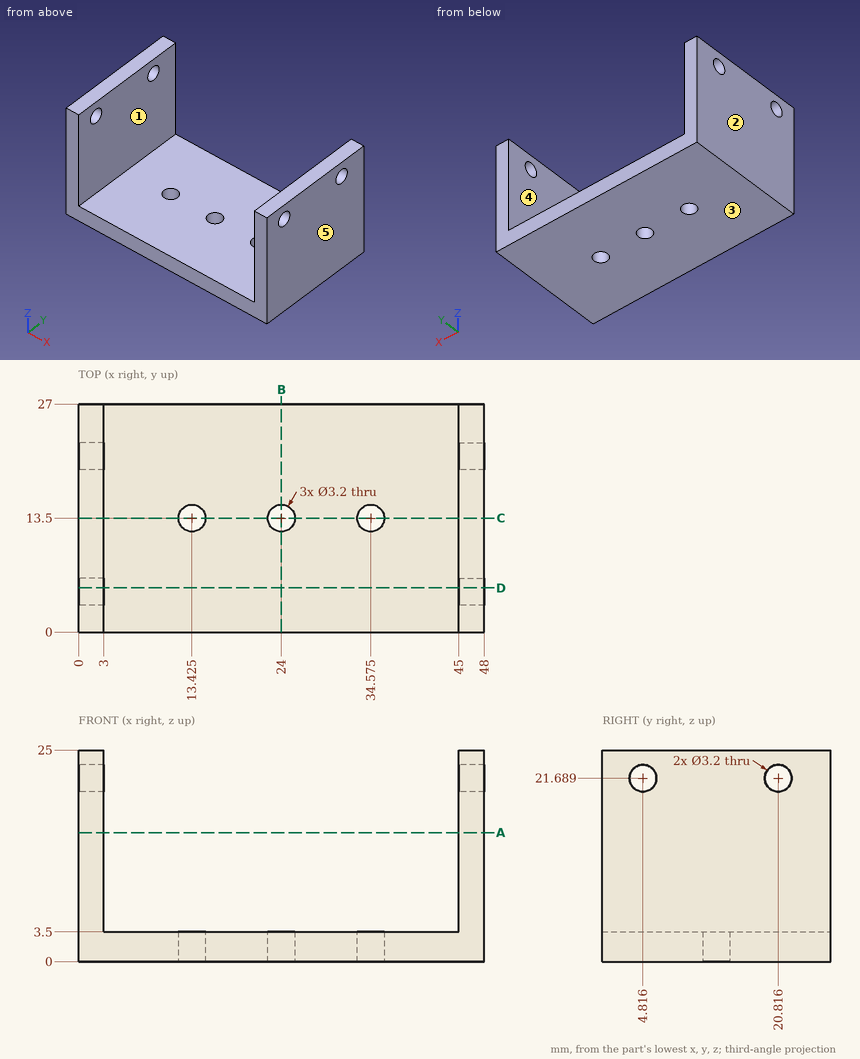
The drawing under review shows one solid part. Ordinate dimensions are in mm from its lowest x, y, z. A direction names the side the tool comes from. Give positions to 0.01 mm unless a question says otherwise; leave off trailing zeros. Loops run counter-clockwise (first coordinate to the right, second up) from the corner with the lowest first, then second, coordinate; pieces in that order, holes last. Notation, with made-up numbers: M 26.5,-9 L 41.5,-9 A9 ccw 41.5,-5 Z; hole C -4,79 d6. An arc over 180 degrees is marked long. Return JSON: item names as keys, results as strings. Group by question number.
Item 1: We need section D-D (y = 5.25). Give the boundary of the cut face in (x, z).
Item 2: We need section C-C (y = 13.5). Give the boundary of the cut face in (x, z) (1 decimal).
Item 3: Insertion check: pin 1 Ø3 at (y, z) = (20.82, 21.69) entering from +X; pin 2 Ø13.5 at (x, y) = (31, 9) entering from +Z. Each pin has a flat end and moves straight along its axis. Give the tip position at first contact, or say it passes through.
Item 4: For probe 1 along X at (y, z) = (15, 9.5); probe 2 along Z at (x, y) = (7, 25); probe 3 along Y at (x, z) = (24, 1.4), list the stretches that pass through material, from the lowest coordinate up.
Item 5: Tool access review of the marked faces 4 and 5: name each direction out of +Z, -Z, +X, -X, +Y, -Y from which nothing blocks a thin tool from reaching the whole face with its end or side.
Item 6: We need section B-B (x = 24). Give the boundary of the cut face in (y, z), and give its area (3 significant figures).
Item 7: We need section A-A (z = 15.25). Give the boundary of the cut face in (x, y).
Item 8: Mouldability with a two-part tool opening along X and no side actions: class the marked faces 1, 2 and 3 as released by +X, released by -X, zero draft, split by the parting line, or undercut.
Output:
{
 "1": {"outline": "M 0,0 L 48,0 L 48,20.15 L 45,20.15 L 45,3.5 L 3,3.5 L 3,20.15 L 0,20.15 Z; M 0,23.23 L 3,23.23 L 3,25 L 0,25 Z; M 45,23.23 L 48,23.23 L 48,25 L 45,25 Z"},
 "2": {"outline": "M 0,0 L 11.8,0 L 11.8,3.5 L 3,3.5 L 3,25 L 0,25 Z; M 15,0 L 22.4,0 L 22.4,3.5 L 15,3.5 Z; M 25.6,0 L 33,0 L 33,3.5 L 25.6,3.5 Z; M 36.2,0 L 48,0 L 48,25 L 45,25 L 45,3.5 L 36.2,3.5 Z"},
 "3": {"pin 1": "passes through", "pin 2": "stops at z = 3.5"},
 "4": {"probe 1": "x = 0 to 3, 45 to 48", "probe 2": "z = 0 to 3.5", "probe 3": "y = 0 to 11.9, 15.1 to 27"},
 "5": {"face 4": "+Z, +Y, -Y", "face 5": "+Z, -Z, +X, +Y, -Y"},
 "6": {"outline": "M 0,0 L 11.9,0 L 11.9,3.5 L 0,3.5 Z; M 15.1,0 L 27,0 L 27,3.5 L 15.1,3.5 Z", "area": "83.3 mm^2"},
 "7": {"outline": "M 0,0 L 3,0 L 3,27 L 0,27 Z; M 45,0 L 48,0 L 48,27 L 45,27 Z"},
 "8": {"face 1": "undercut", "face 2": "released by -X", "face 3": "zero draft"}
}
